Could you check a few things on this model? Use its own coordinates, in mm. Face numbers are marked on the shaded views. A direction names the side the tool comes from. Give positions to 0.01 mm unless a question says otherwise; leave off trailing zeros. Write each loop counter-clockwise with the first axis right and the second up, starting at its lowest first coordinate (ties: lowest second). Pieces come first, ordered by that corner, then holes. Notation, with made-up numbers: M 59.5,71 L 68.5,71 A13 cw 68.5,89 Z; hole C 78.5,40 d8. An arc over 180 degrees is marked long. One line per item, written item: value.
```python
from build123d import *

# Parameters (mm, degrees)
SKETCH1_W           = 48
SKETCH1_H           = 30
BOSS_EXTRUDE1_DEPTH = 10
SKETCH2_W           = 10
SKETCH2_H           = 3
CUT_EXTRUDE1_DEPTH  = 1.5
SKETCH3_W           = 48
SKETCH3_H           = 30
SKETCH3_R           = 1.45
BOSS_EXTRUDE2_DEPTH = 3
SKETCH4_W           = 20
SKETCH4_H           = 30
SKETCH4_R           = 1.45
BOSS_EXTRUDE3_DEPTH = 20
SKETCH5_R           = 6.875
CUT_EXTRUDE2_DEPTH  = 35
FILLET1_R           = 5
CHAMFER1_SIZE       = 8.5


# Some blends are built 0.0001 mm under size
with BuildPart() as part:
    # Sketch1 → Boss-Extrude1 (new body)
    with BuildSketch(Plane.XY):
        with Locations((21, 12)):
            Rectangle(SKETCH1_W, SKETCH1_H)
        Polygon((-0.5, 24.5), (16, 24.5), (16, 21.5), (26, 21.5), (26, 24.5), (42.5, 24.5), (42.5, -0.5), (26, -0.5), (26, 2.5), (16, 2.5), (16, -0.5), (-0.5, -0.5), align=None, mode=Mode.SUBTRACT)
    extrude(amount=BOSS_EXTRUDE1_DEPTH)

    # Sketch2 → Cut-Extrude1 (cut)
    with BuildSketch(Plane.XY.offset(10)):
        with Locations((21, 1)):
            Rectangle(SKETCH2_W, SKETCH2_H)
        with Locations((21, 23)):
            Rectangle(SKETCH2_W, SKETCH2_H)
    extrude(amount=-CUT_EXTRUDE1_DEPTH, mode=Mode.SUBTRACT)

    # Sketch3 → Boss-Extrude2 (add)
    with BuildSketch(Plane(origin=(0, 0, 0), x_dir=(-1, 0, 0), z_dir=(0, 0, -1))):
        with Locations((-21, 12)):
            Rectangle(SKETCH3_W, SKETCH3_H)
        with Locations((-40, 22)):
            Circle(SKETCH3_R, mode=Mode.SUBTRACT)
        with Locations((-40, 2)):
            Circle(SKETCH3_R, mode=Mode.SUBTRACT)
        with Locations((-2, 22)):
            Circle(SKETCH3_R, mode=Mode.SUBTRACT)
        with Locations((-2, 2)):
            Circle(SKETCH3_R, mode=Mode.SUBTRACT)
    extrude(amount=BOSS_EXTRUDE2_DEPTH)

    # Sketch4 → Boss-Extrude3 (add)
    with BuildSketch(Plane(origin=(0, 0, -3), x_dir=(-1, 0, 0), z_dir=(0, 0, -1))):
        with Locations((-35, 12)):
            Rectangle(SKETCH4_W, SKETCH4_H)
        with Locations((-40, 22)):
            Circle(SKETCH4_R, mode=Mode.SUBTRACT)
        with Locations((-40, 2)):
            Circle(SKETCH4_R, mode=Mode.SUBTRACT)
    extrude(amount=BOSS_EXTRUDE3_DEPTH)

    # Sketch5 → Cut-Extrude2 (cut)
    with BuildSketch(Plane(origin=(0, 27, 0), x_dir=(1, 0, 0), z_dir=(0, 1, 0))):
        with Locations(Location((35, 13, 0), (0, 0, 270))):
            Circle(SKETCH5_R)
    extrude(amount=-CUT_EXTRUDE2_DEPTH, mode=Mode.SUBTRACT)

    # Fillet1
    # the kernel refuses this fillet: 5 mm, written as the material it adds along each edge
    with BuildSketch(Plane(origin=(25, 27, -3), x_dir=(-1, 0, 0), z_dir=(0, -1, 0))) as fillet1_piece_1:
        with BuildLine():
            CenterArc((FILLET1_R, FILLET1_R), FILLET1_R, 180, 90)
            Line((0, FILLET1_R), (0, 0))
            Line((0, 0), (FILLET1_R, 0))
        make_face()
    extrude(amount=30)
    # the kernel refuses this fillet: 5 mm, written as the material it takes off along each edge
    with BuildSketch(Plane(origin=(45, -15.5, -23), x_dir=(0, 0, 1), z_dir=(0, 1, 0)), Plane(origin=(-3, 39.5, -3), x_dir=(0, 0, 1), z_dir=(0, -1, 0))) as fillet1_2_piece_1:
        with BuildLine():
            CenterArc((FILLET1_R, -FILLET1_R), FILLET1_R, 90, 90)
            Line((0, -FILLET1_R), (0, 0))
            Line((0, 0), (FILLET1_R, 0))
        make_face()
    extrude(amount=55, mode=Mode.SUBTRACT)
    with BuildSketch(Plane(origin=(25, 39.5, -23), x_dir=(1, 0, 0), z_dir=(0, -1, 0))) as fillet1_2_piece_2:
        with BuildLine():
            CenterArc((FILLET1_R, FILLET1_R), FILLET1_R, 180, 90)
            Line((0, FILLET1_R), (0, 0))
            Line((0, 0), (FILLET1_R, 0))
        make_face()
    extrude(amount=55, mode=Mode.SUBTRACT)

    # Chamfer1
    chamfer1_edges = [part.edges().sort_by_distance(p)[0] for p in [
        (21, 2.5, 0),
    ]]
    chamfer(chamfer1_edges, length=CHAMFER1_SIZE - 0.0001)  # a hair under: the kernel refuses the full size


solid = part.part
```
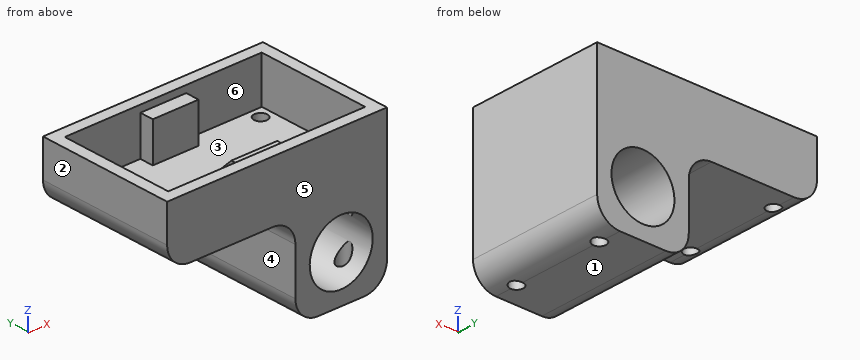
1) If we section it at C-C, the plane y = 19: Write out the boundary of the cut face in (x, z) (3 decimals), then the cut area to 3 significant figures.
Outcome:
outline: M -3,2 A5 ccw 2,-3 L 20,-3 A5 cw 25,-8 L 25,-18 A5 ccw 30,-23 L 40,-23 A5 ccw 45,-18 L 45,10 L 42.5,10 L 42.5,0 L -0.5,0 L -0.5,10 L -3,10 Z; hole C 35,-13 d13.75
area: 435 mm^2
2) If we section it at A-A, the plane z = -13: Write out the boundary of the cut face in (x, y) (3 decimals), then the cut area to 4 significant figures.
Outcome:
outline: M 25,-3 L 28.125,-3 L 28.125,27 L 25,27 Z; M 41.875,-3 L 45,-3 L 45,27 L 41.875,27 Z
area: 187.5 mm^2
3) Please list where these lines run through material, in increasing order: L1, parallel to X at y = 2.5, z = 2.5; L2, parallel to Y at x = 40, z = -18.5; L3, parallel to X at y = 9, z = -13 (3 decimals). Write a range as from..to.
Outcome:
L1: x = -3..-0.5, 16..26, 42.5..45
L2: y = -3..0.55, 3.45..20.55, 23.45..27
L3: x = 25..28.125, 41.875..45
4) If we section it at D-D, the plane x = 15: Write out the boundary of the cut face in (y, z), then the cut area to 3 significant figures.
Outcome:
outline: M -3,-3 L 27,-3 L 27,10 L 24.5,10 L 24.5,0 L -0.5,0 L -0.5,10 L -3,10 Z
area: 140 mm^2
5) If we section it at B-B, the plane x = 35: Write out the boundary of the cut face in (y, z) (3 decimals), then the cut area to 4 significant figures.
Outcome:
outline: M -3,-23 L 27,-23 L 27,-19.875 L -3,-19.875 Z; M -3,-6.125 L 27,-6.125 L 27,10 L 24.5,10 L 24.5,0 L -0.5,0 L -0.5,10 L -3,10 Z
area: 327.5 mm^2
6) On a 3-axis mill with a long thin cutter (end or side, diameter ignored), from which of +Z, -Z, +X, -X, +Y, -Y can I reach the whole of each face in a straight line? I mean the marked faces 4, 5 and 6. Say none if no direction works.
Outcome:
face 4: -Z, -X, +Y, -Y
face 5: +Z, -Z, +X, -X, -Y
face 6: +Z
7) We'd pull the mould along X, two halves only. Please class the marked faces 1, 2 and 3: pulls with the +X half, pulls with the -X half, needs draft (parallel to the pull), parting line crosses it, or undercut.
Outcome:
face 1: needs draft
face 2: pulls with the -X half
face 3: undercut
8) I'm going to push flat-ended pins straight in: pin 1 (1 mm diameter, centred on y = 11, z = -1, fed in from -X); pin 2 (11 mm diameter, centred on y = 10, z = -12, fed in from -X); pin 3 (7.5 mm diameter, centred on x = 27, y = 17, fed in from +Z); pin 4 (1.7 mm diameter, centred on x = 40, y = 22, fed in from -Z). Where does each tip first touch, or does it pass through?
Outcome:
pin 1: stops at x = -2.33
pin 2: stops at x = 24.77
pin 3: stops at z = 0
pin 4: passes through
